Can you work these out from the drawing? Everything is in mm from the part's minimum corner. A direction names the side the tool comes from. Coordinates: 2 decimals unless noted, no trailing zeros. Loops run counter-clockwise (first coordinate to the right, second up) from the corner with the lowest first, then second, coordinate; pieces in that order, holes last. Notation, with made-up numbers: (15.25, 34) -> (36.25, 34) arc R37 ccw to (36.25, 73) -> close; hole circle Ø7 at (-3.75, -22). An arc over 180 degrees is marked (long way). Put each result on its own line as item: value. Start each with the question number.
Item 1: If we section it at D-D on x = 38.5: Please give me the cut outline in (y, z) (3 decimals).
Item 2: For the marked faces 1, 2, 3, 4 and 5, which set-ups out of +Z, -Z, +X, -X, +Y, -Y let a thin tool reach every point of the face, with its end or its side?
Item 3: Please list where these lines run through material, in increasing order: L1, parallel to Y at x = 3.81, z = 1.2 (3 decimals); L2, parallel to X at y = 20, z = 2.75; L3, parallel to Z at x = 56, y = 35. Write a range as from..to.
Item 4: Will these pins go through, and if not, where does the flat tip stop? P1, Ø1.5, axis at y = 15.5, z = 10, coming from the -X side; P2, Ø4, axis at x = 81.28, y = 62.865, coming from the +Z side; P3, Ø1.8, axis at x = 3.81, y = 62.865, coming from the -Z side; P4, Ø7.5, axis at x = 29.5, z = 7.5, coming from the +Y side.
Item 5: If we section it at A-A on z = 12.75: Please give me the cut outline in (x, y), plus the area to 3 significant figures.
Item 6: If we section it at B-B on x = 58.5: Please give me the cut outline in (y, z) (3 decimals), plus the area to 3 significant figures.
Item 7: If we section it at C-C on y = 55: Please give me the cut outline in (x, z).
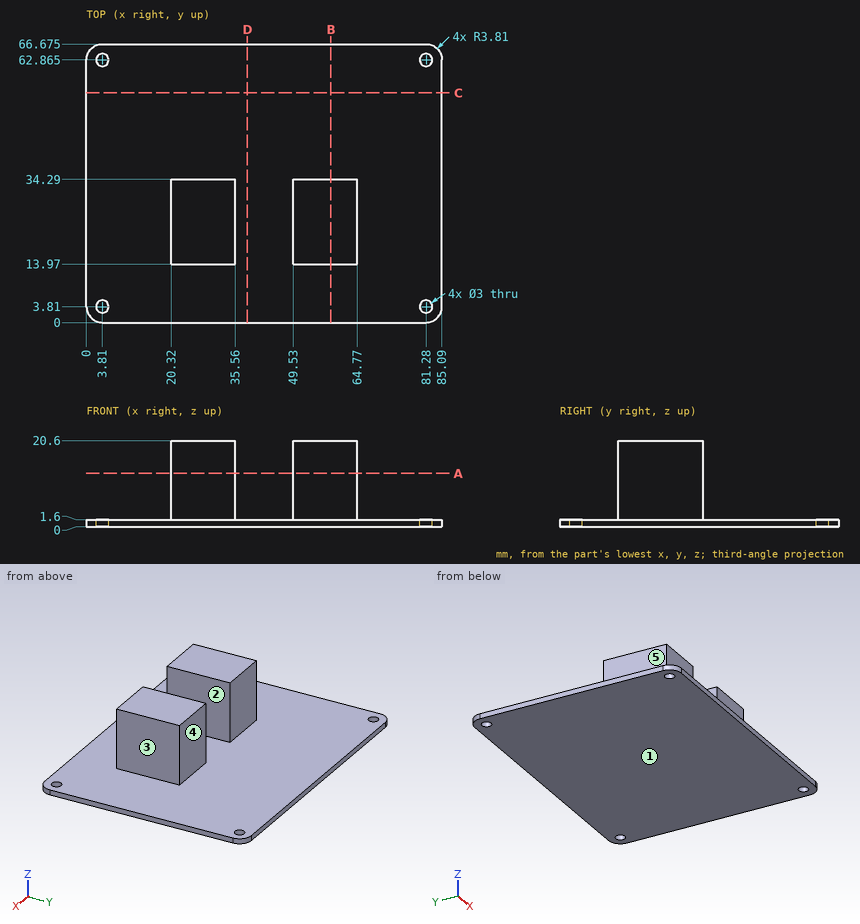
Solutions:
1. outline: (0, 0) -> (66.675, 0) -> (66.675, 1.6) -> (0, 1.6) -> close
2. face 1: -Z, +X, -X, +Y, -Y
2. face 2: +Z, +Y, -Y
2. face 3: +Z, +X, +Y, -Y
2. face 4: +Z, +X, -X, +Y
2. face 5: +Z, -X, +Y, -Y
3. L1: 0..2.31, 5.31..61.365, 64.365..66.675
3. L2: 20.32..35.56, 49.53..64.77
3. L3: 0..1.6
4. P1: x = 20.32
4. P2: z = 1.6
4. P3: through
4. P4: y = 34.29
5. outline: (20.32, 13.97) -> (35.56, 13.97) -> (35.56, 34.29) -> (20.32, 34.29) -> close; (49.53, 13.97) -> (64.77, 13.97) -> (64.77, 34.29) -> (49.53, 34.29) -> close
5. area: 619 mm^2
6. outline: (0, 0) -> (66.675, 0) -> (66.675, 1.6) -> (34.29, 1.6) -> (34.29, 20.6) -> (13.97, 20.6) -> (13.97, 1.6) -> (0, 1.6) -> close
6. area: 493 mm^2
7. outline: (0, 0) -> (85.09, 0) -> (85.09, 1.6) -> (0, 1.6) -> close
